from build123d import *

# Parameters (mm, degrees)
SKETCH1_W           = 270
SKETCH1_H           = 110
BOSS_EXTRUDE1_DEPTH = 4
SKETCH9_R           = 3
SKETCH9_R_2         = 2
SKETCH9_R_3         = 1.5
SKETCH9_W           = 10
SKETCH9_H           = 52.992911327
CUT_EXTRUDE1_DEPTH  = 146.828666592


with BuildPart() as part:
    # Sketch1 → Boss-Extrude1 (new body)
    with BuildSketch(Plane.XY):
        Rectangle(SKETCH1_W, SKETCH1_H)
    extrude(amount=BOSS_EXTRUDE1_DEPTH)

    # Sketch9 → Cut-Extrude1 (cut, through all)
    with BuildSketch(Plane(origin=(0, 0, 0), x_dir=(-1, 0, 0), z_dir=(0, 0, -1))):
        with Locations((-120, 46)):
            Circle(SKETCH9_R)
        with Locations((-127, -46)):
            Circle(SKETCH9_R)
        with Locations((120, 46)):
            Circle(SKETCH9_R)
        with Locations((127, -46)):
            Circle(SKETCH9_R)
        with Locations((-4.074540436, -6)):
            Circle(SKETCH9_R_2)
        with Locations((4.925459564, -17)):
            Circle(SKETCH9_R_2)
        with Locations((27.925459564, -17)):
            Circle(SKETCH9_R_2)
        with Locations((37.925459564, -6.5)):
            Circle(SKETCH9_R_2)
        with Locations((37.925459564, 18.5)):
            Circle(SKETCH9_R_2)
        with Locations((18.425459564, 28.5)):
            Circle(SKETCH9_R_3)
        with Locations((-9.574540436, 28.503544336)):
            Rectangle(SKETCH9_W, SKETCH9_H)
    extrude(amount=-CUT_EXTRUDE1_DEPTH, mode=Mode.SUBTRACT)


solid = part.part
The listing builds one solid part. Answer for the finished solid, in the listing's coordinates (mm). Give positions to 0.01 mm unless a question says otherwise; leave off trailing zeros. Loops run counter-clockwise (first coordinate to the right, second up) from the corner with the lowest first, then second, coordinate; pieces in that order, holes last. Notation, with made-up numbers: M 9.5,7 L 66.5,7 A15 ccw 66.5,31 Z; hole C 66.5,52.25 d9. An arc over 180 degrees is marked long. Answer as CSV lines item,"result".
Item 1: The part is cut by section D-D (y = -46). Give the vertices of the cut face in (x, z).
Values follow:
outline,"M -135,0 L -130,0 L -130,4 L -135,4 Z; M -124,0 L 124,0 L 124,4 L -124,4 Z; M 130,0 L 135,0 L 135,4 L 130,4 Z"
Item 2: The part is cut by section A-A (y = 46). Give the vertices of the cut face in (x, z).
Values follow:
outline,"M -135,0 L -123,0 L -123,4 L -135,4 Z; M -117,0 L 4.57,0 L 4.57,4 L -117,4 Z; M 14.57,0 L 117,0 L 117,4 L 14.57,4 Z; M 123,0 L 135,0 L 135,4 L 123,4 Z"
Item 3: The part is cut by section C-C (x = -127). Give the vertices of the cut face in (y, z).
Values follow:
outline,"M -55,0 L -49,0 L -49,4 L -55,4 Z; M -43,0 L 55,0 L 55,4 L -43,4 Z"
Item 4: Straight lines are drawn through the part: line 1 along Y through (x, z) = (-38, 2.7); line 2 along X through (y, z) = (19, 2.95); line 3 along Y through (x, z) = (-120, 1.8). For each, find the intervals that lie inside material, in ascending order. Write a range as [from, to].
Values follow:
line 1,"y = [-55, -8.5], [-4.5, 16.5], [20.5, 55]"
line 2,"x = [-135, -39.86], [-35.99, 4.57], [14.57, 135]"
line 3,"y = [-55, 43], [49, 55]"
Item 5: The mould has two halves that part along X. Classify faces 1 (the cylindrical face through (124.14, -45.1, 1.97)), 2 (the flat face through (-2, 1, 4)), 3 (the cylindrical face through (-122.86, 46.9, 1.97)): released by +X, released by -X, zero draft, split by the parting line, or undercut.
Values follow:
face 1,"undercut"
face 2,"zero draft"
face 3,"undercut"
Item 6: The part is cut by section B-B (y = 9). Give the vertices of the cut face in (x, z).
Values follow:
outline,"M -135,0 L 4.57,0 L 4.57,4 L -135,4 Z; M 14.57,0 L 135,0 L 135,4 L 14.57,4 Z"
Item 7: Given pin 1 Ø7 at (x, y) = (127, -46) entering from -Z, flat-ended and moving along its own axis, determine where the tip first touches the part or whether it passes through.
Values follow:
pin 1,"stops at z = 0"
